For this review, take the finished solid that the model builds, in its own axes (mm). Face numbers are marked on the shaded views. A direction names the side the tool comes from. Coordinates: 2 decimals unless noted, no trailing zeros. Write each loop counter-clockwise with the first axis right and the second up, starting at its lowest first coordinate (ties: lowest second). Pieces come first, ordered by that corner, then holes. Notation, with made-up numbers: M 21,60 L 78,60 A25 ccw 78,96 Z; hole C 40,54.25 d10. An arc over 180 degrees is marked long. One line per question, with ' | ' between items.
from build123d import *

# Parameters (mm, degrees)
IZIM1_W                     = 350
IZIM1_H                     = 348
IZIM1_R                     = 12.5
Y_KSEKLIK_EKSTR_ZYON4_DEPTH = 344
BO_ALTMA2_T                 = -8


with BuildPart() as part:
    # Çizim1 → Yükseklik-Ekstrüzyon4 (new body)
    with BuildSketch(Plane.XY):
        with Locations((-50, -6)):
            Rectangle(IZIM1_W, IZIM1_H)
        Circle(IZIM1_R, mode=Mode.SUBTRACT)
        with Locations((-108.440540321, 32.652897497)):
            Circle(IZIM1_R, mode=Mode.SUBTRACT)
        with Locations((-120.297461902, -75.448794953)):
            Circle(IZIM1_R, mode=Mode.SUBTRACT)
    extrude(amount=-Y_KSEKLIK_EKSTR_ZYON4_DEPTH)

    # İç Boşaltma2
    bo_altma2_openings = [part.faces().sort_by_distance(p)[0] for p in [
        (12.5, 0, -344),
        (-50, 168, -172),
        (-107.797461902, -75.448794953, -344),
        (-95.940540321, 32.652897497, -344),
    ]]
    offset(amount=BO_ALTMA2_T, openings=bo_altma2_openings, kind=Kind.INTERSECTION)


solid = part.part
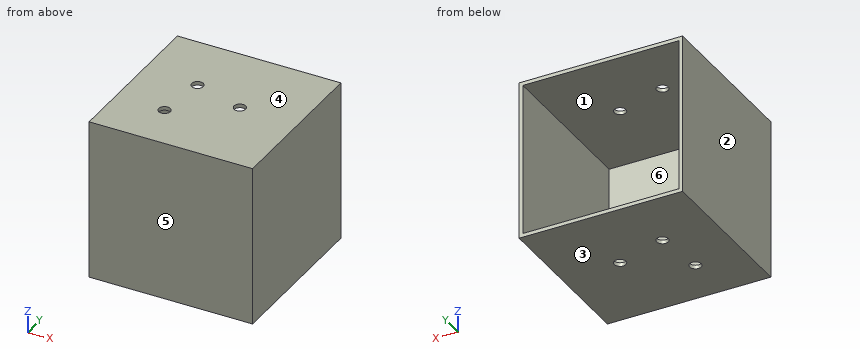
1. Clearance check with a flat-ended pin moving along its axis: P1, Ø12, axis at x = -125, z = -114, coming from the +Y side. State where the tip first meets the part, or that it passes through.
Computed values:
P1: stops at y = -172
2. Take a section at A-A on y = 0. State the section outline as (x, z) points, plus the area to 3 significant figures.
Computed values:
outline: M -225,-344 L -12.5,-344 L -12.5,-336 L -217,-336 L -217,-8 L -12.5,-8 L -12.5,0 L -225,0 Z; M 12.5,-344 L 125,-344 L 125,0 L 12.5,0 L 12.5,-8 L 117,-8 L 117,-336 L 12.5,-336 Z | area: 10,400 mm2
3. Draft analysis for pull direction Z (two halves, no side actions). For the marked faces 1, 2, 3 and 4, state which applies: pulls with the +Z half, pulls with the -Z half, needs draft (parallel to the pull), parting line crosses it, or undercut.
Computed values:
face 1: undercut | face 2: needs draft | face 3: pulls with the -Z half | face 4: pulls with the +Z half
4. Take a section at B-B on x = 0. State the section outline as (y, z) points, plus the area to 3 significant figures.
Computed values:
outline: M -180,-344 L -12.5,-344 L -12.5,-336 L -172,-336 L -172,-8 L -12.5,-8 L -12.5,0 L -180,0 Z; M 12.5,-344 L 168,-344 L 168,-336 L 12.5,-336 Z; M 12.5,-8 L 168,-8 L 168,0 L 12.5,0 Z | area: 7,790 mm2
5. Machinability: for the marked faces 5 and 6, which of the approach directions +Z, -Z, +X, -X, +Y, -Y give a long, thin tool a straight path to every point of the face, cutting with its end or side? Answer none if there is none.
Computed values:
face 5: +Z, -Z, +X, -X, -Y | face 6: +Y
6. Take a section at C-C on y = -51.5. State the section outline as (x, z) points, plus the area to 3 significant figures.
Computed values:
outline: M -225,-344 L 125,-344 L 125,0 L -225,0 Z; hole M -217,-336 L 117,-336 L 117,-8 L -217,-8 Z | area: 10,800 mm2
7. For line 1 along Z through (x, y) = (-59, -30); line 2 along X through (y, z) = (-20.5, -60.5); line 3 along Y through (x, z) = (0, -339), list the stretches that pass through material, from the lowest coordinate up.
Computed values:
line 1: z = -344 to -336, -8 to 0 | line 2: x = -225 to -217, 117 to 125 | line 3: y = -180 to -12.5, 12.5 to 168
8. Take a section at D-D on z = -242.5. State the section outline as (x, y) points, plus the area to 3 significant figures.
Computed values:
outline: M -225,-180 L 125,-180 L 125,168 L 117,168 L 117,-172 L -217,-172 L -217,168 L -225,168 Z | area: 8,240 mm2
